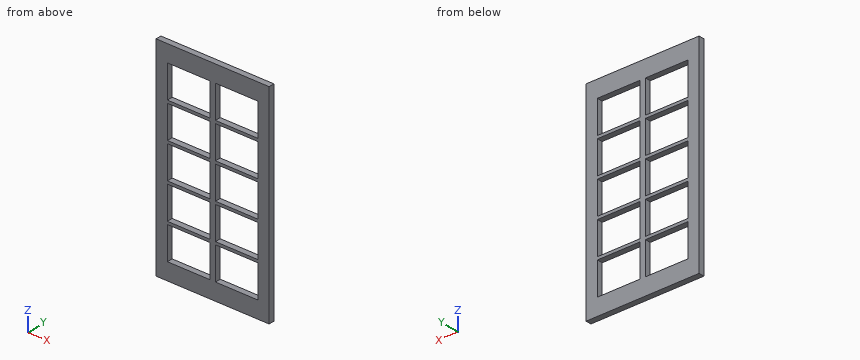
```python
from build123d import *

# Parameters (mm, degrees)
F0_W     = 1016
F0_H     = 1879.6
F1_DEPTH = 50.8
F2_W     = 381
F2_H     = 294.64
F3_DEPTH = 50.801


with BuildPart() as f1:
    # F0 (on Front) → F1 (new body)
    with BuildSketch(Plane.XZ):
        Rectangle(F0_W, F0_H)
    extrude(amount=F1_DEPTH)

    # F2 (on face) → F3 (cut, through all)
    with BuildSketch(Plane.XZ.offset(50.8)):
        with Locations((-215.9, 640.08)):
            Rectangle(F2_W, F2_H)
        with Locations((-215.9, 320.04)):
            Rectangle(F2_W, F2_H)
        with Locations((-215.9, 0)):
            Rectangle(F2_W, F2_H)
        with Locations((-215.9, -320.04)):
            Rectangle(F2_W, F2_H)
        with Locations((-215.9, -640.08)):
            Rectangle(F2_W, F2_H)
        with Locations((215.9, 320.04)):
            Rectangle(F2_W, F2_H)
        with Locations((215.9, 640.08)):
            Rectangle(F2_W, F2_H)
        with Locations((215.9, 0)):
            Rectangle(F2_W, F2_H)
        with Locations((215.9, -320.04)):
            Rectangle(F2_W, F2_H)
        with Locations((215.9, -640.08)):
            Rectangle(F2_W, F2_H)
    extrude(amount=-F3_DEPTH, mode=Mode.SUBTRACT)


solid = f1.part
```
Geometry: final body of the model. Coordinates: model frame, mm. Give positions to 0.01 mm unless a question says otherwise; leave off trailing zeros. Loops run counter-clockwise (first coordinate to the right, second up) from the corner with the lowest first, then second, coordinate; pieces in that order, holes last. Notation, with made-up numbers: (0, 86) - (24, 86) arc R23 ccw to (24, 102) - close; hole circle Ø4 at (24.5, 66). An arc over 180 degrees is marked (long way). Answer as CSV lines item,"result". Start each with the question number.
(1) Ray query, line 1 along Z through (x, y) = (-180, -28); line 2 along X through (y, z) = (-38, 719.5). Return the intervals inside material, ascending. Write a range as [from, to].
(2) Section query B-B (x = -46). Output: boundary loops of the cut face in (y, z).
(3) Section query C-C (y = -26). Give the number of separate pieces and of enclosed holes in the cut face, and give its area (3 significant figures).
(4) Section query A-A (z = -676.5). Output: boundary loops of the cut face in (x, y), and give its area (3 significant figures).
Worked answers:
1,line 1,"z = [-939.8, -787.4], [-492.76, -467.36], [-172.72, -147.32], [147.32, 172.72], [467.36, 492.76], [787.4, 939.8]"
1,line 2,"x = [-508, -406.4], [-25.4, 25.4], [406.4, 508]"
2,outline,"(-50.8, -939.8) - (0, -939.8) - (0, -787.4) - (-50.8, -787.4) - close; (-50.8, -492.76) - (0, -492.76) - (0, -467.36) - (-50.8, -467.36) - close; (-50.8, -172.72) - (0, -172.72) - (0, -147.32) - (-50.8, -147.32) - close; (-50.8, 147.32) - (0, 147.32) - (0, 172.72) - (-50.8, 172.72) - close; (-50.8, 467.36) - (0, 467.36) - (0, 492.76) - (-50.8, 492.76) - close; (-50.8, 787.4) - (0, 787.4) - (0, 939.8) - (-50.8, 939.8) - close"
3,separate pieces,"1"
3,enclosed holes,"10"
3,area,"787,000 mm^2"
4,outline,"(-508, -50.8) - (-406.4, -50.8) - (-406.4, 0) - (-508, 0) - close; (-25.4, -50.8) - (25.4, -50.8) - (25.4, 0) - (-25.4, 0) - close; (406.4, -50.8) - (508, -50.8) - (508, 0) - (406.4, 0) - close"
4,area,"12,900 mm^2"
